Build history of the part. All positions in model axes, mm. A direction names the side the tool comes from. Coordinates: 2 decimals unless noted, no trailing zeros. Loops run counter-clockwise (first coordinate to the right, second up) from the corner with the lowest first, then second, coordinate; pieces in that order, holes last.
(1) Two-plate mould, pull along X, no slides. Class faces 4 (the face through (9.818, 14.048, -35.464)), 5 (the face through (20, 2, 31)), 6 (the face through (27, 43, 36)), 7 (the face through (12.93, 1.48, -31.5)): pulls with the +X half, pulls with the -X half, needs draft (parallel to the pull), parting line crosses it, or undercut.
(2) Slice it at C-C (y = 40). Give the cut face in (x, z).
(3) Wall check: L1, parallel to Y at x = 18, z = -18.5; L2, parallel to Z at x = 15, y = 14.5; L3, parallel to Y at x = 18.5, z = -20. Give the ranges that are in metal, low to high.
(4) Flat gauge pins, fed straight in: P1, Ø12, axis at y = 30, z = 1, coming from the +X side; P2, Ø6, axis at y = 26.5, z = -20, coming from the -X side; P3, Ø3.5, axis at y = 1.5, z = 6, coming from the -X side. Where does each tip first touch, or does it go through?
(5) Slice it at B-B (z = 3). Give the cut face in (x, y).
(6) Tool access for faces 1 (the face through (14.281, 21.777, -31.07)), 2 (the face through (20, 2, -31)), 3 (the face through (23.281, 37.366, -31.07)): list every direction of +Z, -Z, +X, -X, +Y, -Y with a clear straight run to the whole face (end or side of a thin tool).
(7) Slice it at A-A (z = 30). Give the cut face in (x, y).
from build123d import *

# Parameters (mm, degrees)
EXTRUDE_1_DEPTH      = 36
EXTRUDE_1_DEPTH_BACK = 36
EXTRUDE_2_DEPTH      = 60
SKETCH_4_R           = 1.5
SKETCH_4_W           = 10
SKETCH_4_H           = 18
CUT_EXTRUDE_1_DEPTH  = 6
CUT_EXTRUDE_3_DEPTH  = 14
SKETCH_9_R           = 1.5
CUT_EXTRUDE_5_DEPTH  = 6
CUT_EXTRUDE_6_DEPTH  = 3
FILLET_1_R           = 1
CHAMFER_1_SIZE       = 10


with BuildPart() as part:
    # 草图2 → 凸台-拉伸1 (new, two sides: drawn at the far end of the back side and taken through both)
    with BuildSketch(Plane.XY.offset(-EXTRUDE_1_DEPTH_BACK)):
        Polygon((0, 0), (28.5, 49.363448016), (31.098076211, 47.863448016), (5.196152423, 3), (25, 3), (25, 0), align=None)
    extrude(amount=EXTRUDE_1_DEPTH + EXTRUDE_1_DEPTH_BACK)

    # 草图3 → 凸台-拉伸2 (add)
    with BuildSketch(Plane.XY.offset(36)):
        Polygon((13.196152423, 16.856406461), (14.696152423, 19.454482672), (24.196152423, 3), (21.196152423, 3), align=None)
    extrude(amount=-EXTRUDE_2_DEPTH)

    # 草图4 → 切除-拉伸1 (cut)
    with BuildSketch(Plane(origin=(0, 0, 0), x_dir=(0, 0, 1), z_dir=(-0.8660254037844365, 0.500000000000004, 0))):
        with Locations(Location((34, 53.25, 0), (0, 0, 270))):
            Circle(SKETCH_4_R)
        with Locations(Location((34, 16.75, 0), (0, 0, 90))):
            Circle(SKETCH_4_R)
        with Locations(Location((-34, 16.75, 0), (0, 0, 270))):
            Circle(SKETCH_4_R)
        with Locations(Location((-34, 53.25, 0), (0, 0, 90))):
            Circle(SKETCH_4_R)
        with Locations((31, 35)):
            Rectangle(SKETCH_4_W, SKETCH_4_H)
        with Locations((-31, 35)):
            Rectangle(SKETCH_4_W, SKETCH_4_H)
    extrude(amount=-CUT_EXTRUDE_1_DEPTH, mode=Mode.SUBTRACT)

    # 草图6 → 切除-拉伸3 (cut)
    with BuildSketch(Plane.XY.offset(36)):
        Polygon((24.196152423, 3), (14.696152423, 19.454482672), (13.196152423, 16.856406461), (21.196152423, 3), align=None)
    extrude(amount=-CUT_EXTRUDE_3_DEPTH, mode=Mode.SUBTRACT)

    # 草图9 → 切除-拉伸5 (cut)
    with BuildSketch(Plane.XZ):
        with Locations(Location((13, 30, 0), (0, 0, 270))):
            Circle(SKETCH_9_R)
        with Locations(Location((13, -30, 0), (0, 0, 90))):
            Circle(SKETCH_9_R)
        with BuildLine():
            Line((9, -12.5), (9, 12.5))
            ThreePointArc((9, 12.5), (13, 16.5), (17, 12.5))
            Line((17, 12.5), (17, -12.5))
            ThreePointArc((17, -12.5), (13, -16.5), (9, -12.5))
        make_face()
    extrude(amount=-CUT_EXTRUDE_5_DEPTH, mode=Mode.SUBTRACT)

    # 草图11 → 切除-拉伸6 (cut)
    with BuildSketch(Plane(origin=(19.446152423, 11.227241336, 0), x_dir=(0, 0, -1), z_dir=(0.8660254037844374, 0.5000000000000022, 0))):
        with BuildLine():
            Line((-10, 4), (10, 4))
            ThreePointArc((10, 4), (14, 0), (10, -4))
            Line((10, -4), (-10, -4))
            ThreePointArc((-10, -4), (-14, 0), (-10, 4))
        make_face()
    extrude(amount=-CUT_EXTRUDE_6_DEPTH, mode=Mode.SUBTRACT)

    # 圆角1
    # the kernel refuses this fillet: 1 mm, written as the material it takes off along each edge
    with BuildSketch(Plane(origin=(16.848076211, 23.181724008, -36), x_dir=(-0.8660254037844364, 0.500000000000004, 0), z_dir=(-0.5000000000000039, -0.8660254037844364, 0))) as fillet_1_piece_1_section:
        with BuildLine():
            CenterArc((FILLET_1_R, -FILLET_1_R), FILLET_1_R, 90, 90)
            Line((0, -FILLET_1_R), (0, 0))
            Line((0, 0), (FILLET_1_R, 0))
        make_face()
    fillet_1_piece_1 = extrude(amount=25.803847577, mode=Mode.PRIVATE)
    fillet_1_piece_1 = split(fillet_1_piece_1, bisect_by=Plane(origin=(10.79221618, 3, -35.774281329), z_dir=(0, 1, 0)), keep=Keep.TOP, mode=Mode.PRIVATE)
    add(fillet_1_piece_1, mode=Mode.SUBTRACT)
    with BuildSketch(Plane(origin=(3.946152423, 0.834936491, 36), x_dir=(-0.8660254037844366, 0.5000000000000037, 0), z_dir=(0.5000000000000037, 0.8660254037844366, 0))) as fillet_1_piece_2_section:
        with BuildLine():
            CenterArc((FILLET_1_R, -FILLET_1_R), FILLET_1_R, 90, 90)
            Line((0, -FILLET_1_R), (0, 0))
            Line((0, 0), (FILLET_1_R, 0))
        make_face()
    fillet_1_piece_2 = extrude(amount=25.803847577, mode=Mode.PRIVATE)
    fillet_1_piece_2 = split(fillet_1_piece_2, bisect_by=Plane(origin=(10.79221618, 3, 35.774281329), z_dir=(0, 1, 0)), keep=Keep.TOP, mode=Mode.PRIVATE)
    add(fillet_1_piece_2, mode=Mode.SUBTRACT)

    # 倒角1
    chamfer_1_edges = [part.edges().sort_by_distance(p)[0] for p in [
        (25, 1.5, 36),
        (25, 1.5, -36),
    ]]
    chamfer(chamfer_1_edges, length=CHAMFER_1_SIZE)


solid = part.part
Response values:
1. face 4: undercut
1. face 5: pulls with the +X half
1. face 6: needs draft
1. face 7: undercut
2. outline: (23.09, -36) - (26.56, -36) - (26.56, 36) - (23.09, 36) - close
3. L1: y = 0 to 3, 8.54 to 13.73, 25.18 to 31.18
3. L2: z = -24 to 22
3. L3: y = 0 to 3, 7.67 to 12.87, 26.04 to 32.04
4. P1: stops at x = 24.25
4. P2: stops at x = 13.57
4. P3: stops at x = 0
5. outline: (0, 0) - (9, 0) - (9, 3) - (5.2, 3) - (13.2, 16.86) - (15.2, 13.39) - (17.45, 14.69) - (14.7, 19.45) - (31.1, 47.86) - (28.5, 49.36) - close; (17, 0) - (25, 0) - (25, 3) - (24.2, 3) - (21.45, 7.76) - (19.2, 6.46) - (21.2, 3) - (17, 3) - close
6. face 1: -Z, +X, +Y
6. face 2: -Z, +X, -Y
6. face 3: -Z, -X
7. outline: (0, 0) - (11.5, 0) - (11.5, 3) - (5.2, 3) - (15.6, 21.02) - (13, 22.52) - close; (14.5, 0) - (21, 0) - (21, 3) - (14.5, 3) - close; (22, 38.11) - (24.6, 36.61) - (31.1, 47.86) - (28.5, 49.36) - close
